```python
from build123d import *

# Parameters (mm, degrees)
EXTRUDE_1_DEPTH     = 22
EXTRUDE_2_DEPTH     = 21
CUT_EXTRUDE_1_REACH = 66.591
CUT_EXTRUDE_2_DEPTH = 11
FILLET_2_R          = 3
FILLET_3_R          = 4
SKETCH_6_W          = 11
SKETCH_6_H          = 2.5
EXTRUDE_6_DEPTH     = 5
FILLET_4_R          = 5
FILLET_5_R          = 2.5
SKETCH_7_R          = 1.5
CUT_EXTRUDE_3_DEPTH = 16
CUT_EXTRUDE_4_DEPTH = 11
CUT_EXTRUDE_5_DEPTH = 0.5
FILLET_7_R          = 1.5
FILLET_8_R          = 1
SKETCH_10_R         = 4.5
EXTRUDE_7_DEPTH     = 8
SKETCH_11_R         = 1.5
CUT_EXTRUDE_6_DEPTH = 3
CUT_EXTRUDE_START   = -3
SKETCH_12_R         = 1.5
CUT_EXTRUDE_7_DEPTH = 3


with BuildPart() as part:
    # Эскиз1 → Бобышка-Вытянуть1 (new, symmetric)
    with BuildSketch(Plane(origin=(0, 0, 0), x_dir=(0, 0, -1), z_dir=(1, 0, 0))):
        Polygon((0, -18), (0, 0), (58, 0), (58, -6), (2, -6), (2, -18), align=None)
    extrude(amount=EXTRUDE_1_DEPTH, both=True)

    # Эскиз2 → Бобышка-Вытянуть2 (add, symmetric)
    with BuildSketch(Plane(origin=(0, 0, 0), x_dir=(0, 0, -1), z_dir=(1, 0, 0))):
        Polygon((2, -6), (48, -6), (48, -7), (3, -7), (3, -17), (2, -17), align=None)
    extrude(amount=EXTRUDE_2_DEPTH, both=True)

    # Вырез-Вытянуть1: up to this face of the body (flat: up to its plane)
    cut_extrude_1_end = Plane(part.part.faces().sort_by_distance((0, -18, -1))[0])
    # Эскиз3 → Вырез-Вытянуть1 (cut, up to the picked face)
    with BuildSketch(Plane(origin=(0, 0, 0), x_dir=(1, 0, 0), z_dir=(0, 1, 0)), mode=Mode.PRIVATE) as cut_extrude_1_sk1:
        Polygon((-20, 58), (-22, 58), (-22, 0), align=None)
    cut_extrude_1_tool1 = split(extrude(cut_extrude_1_sk1.sketch, amount=-CUT_EXTRUDE_1_REACH, mode=Mode.PRIVATE), bisect_by=cut_extrude_1_end, keep=Keep.BOTH, mode=Mode.PRIVATE)
    # Эскиз3 → Вырез-Вытянуть1 (cut, up to the picked face)
    with BuildSketch(Plane(origin=(0, 0, 0), x_dir=(1, 0, 0), z_dir=(0, 1, 0)), mode=Mode.PRIVATE) as cut_extrude_1_sk2:
        Polygon((22, 58), (22, 0), (20, 58), align=None)
    cut_extrude_1_tool2 = split(extrude(cut_extrude_1_sk2.sketch, amount=-CUT_EXTRUDE_1_REACH, mode=Mode.PRIVATE), bisect_by=cut_extrude_1_end, keep=Keep.BOTH, mode=Mode.PRIVATE)
    add(cut_extrude_1_tool1.solids().sort_by(Axis((-21.333333, 0, -38.666667), (0, -1, 0)))[0], mode=Mode.SUBTRACT)
    add(cut_extrude_1_tool2.solids().sort_by(Axis((21.333333, 0, -38.666667), (0, -1, 0)))[0], mode=Mode.SUBTRACT)

    # Эскиз4 → Вырез-Вытянуть2 (cut)
    with BuildSketch(Plane.XZ.offset(6)):
        Polygon((-20.930440129, -2), (-19.344233233, -48), (-20.344827586, -48), (-21.931034483, -2), align=None)
        Polygon((19.344233233, -48), (20.344827586, -48), (21.931034483, -2), (20.930440129, -2), align=None)
    extrude(amount=CUT_EXTRUDE_2_DEPTH, mode=Mode.SUBTRACT)

    # Скругление2
    fillet_2_edges = [part.edges().sort_by_distance(p)[0] for p in [
        (19.344233233, -6.5, -48),
        (-19.344233233, -6.5, -48),
        (-20.91319875, -17, -2.5),
        (20.91319875, -17, -2.5),
    ]]
    fillet(fillet_2_edges, radius=FILLET_2_R)

    # Скругление3
    fillet_3_edges = [part.edges().sort_by_distance(p)[0] for p in [
        (-21.965517241, -18, -1),
        (21.965517241, -18, -1),
    ]]
    fillet(fillet_3_edges, radius=FILLET_3_R)

    # Эскиз6 → Бобышка-Вытянуть6 (add)
    with BuildSketch(Plane.XY):
        with Locations((-16.5, 1.25)):
            Rectangle(SKETCH_6_W, SKETCH_6_H)
        with Locations((16.5, 1.25)):
            Rectangle(SKETCH_6_W, SKETCH_6_H)
    extrude(amount=-EXTRUDE_6_DEPTH)

    # Скругление4
    fillet_4_edges = [part.edges().sort_by_distance(p)[0] for p in [
        (-20.913793103, 0, -31.5),
        (20.913793103, 0, -31.5),
    ]]
    fillet(fillet_4_edges, radius=FILLET_4_R)

    # Скругление5
    fillet_5_edges = [part.edges().sort_by_distance(p)[0] for p in [
        (-16.5, 2.5, -5),
        (-16.5, 2.5, 0),
        (16.5, 2.5, -5),
        (16.5, 2.5, 0),
    ]]
    fillet(fillet_5_edges, radius=FILLET_5_R - 0.0001)  # a hair under: the kernel refuses the full size

    # Эскиз7 → Вырез-Вытянуть3 (cut, symmetric)
    with BuildSketch(Plane(origin=(0, 0, 0), x_dir=(0, 0, -1), z_dir=(1, 0, 0))):
        with Locations((2.5, 0)):
            Circle(SKETCH_7_R)
    extrude(amount=CUT_EXTRUDE_3_DEPTH, both=True, mode=Mode.SUBTRACT)

    # Эскиз8 → Вырез-Вытянуть4 (cut, symmetric)
    with BuildSketch(Plane(origin=(0, 0, 0), x_dir=(0, 0, -1), z_dir=(1, 0, 0))):
        with BuildLine():
            Line((2.5, -2.5), (0, -2.5))
            Line((0, -2.5), (0, 0))
            ThreePointArc((0, 0), (4.267766953, 1.767766953), (2.5, -2.5))
        make_face()
    extrude(amount=CUT_EXTRUDE_4_DEPTH, both=True, mode=Mode.SUBTRACT)

    # Эскиз9 → Вырез-Вытянуть5 (cut)
    with BuildSketch(Plane(origin=(0, 0, -58), x_dir=(-1, 0, 0), z_dir=(0, 0, -1))):
        with BuildLine():
            Line((-14.997028232, -1), (14.997028232, -1))
            add(Edge.make_bspline(
                [(14.997028232, -1), (15.521093765, -1), (16.044951376, -1.104143211), (17.013235139, -1.504981238), (17.457278985, -1.801515154), (18.198254652, -2.542050681), (18.494897371, -2.985758471), (18.895847322, -3.953162299), (19, -4.476479025), (19, -5)],
                knots=[0, 0, 0, 0, 0.25, 0.25, 0.5, 0.5, 0.75, 0.75, 1, 1, 1, 1], degree=3))
            Line((19, -5), (19, -6))
            Line((19, -6), (-19, -6))
            Line((-19, -6), (-19, -5))
            add(Edge.make_bspline(
                [(-14.997028232, -1), (-15.521093765, -1), (-16.044951376, -1.104143211), (-17.013235139, -1.504981238), (-17.457278985, -1.801515154), (-18.198254652, -2.542050681), (-18.494897371, -2.985758471), (-18.895847322, -3.953162299), (-19, -4.476479025), (-19, -5)],
                knots=[0, 0, 0, 0, 0.25, 0.25, 0.5, 0.5, 0.75, 0.75, 1, 1, 1, 1], degree=3))
        make_face()
    extrude(amount=-CUT_EXTRUDE_5_DEPTH, mode=Mode.SUBTRACT)

    # Скругление7
    fillet_7_edges = [part.edges().sort_by_distance(p)[0] for p in [
        (0, -6, -57.5),
    ]]
    fillet(fillet_7_edges, radius=FILLET_7_R)

    # Скругление8
    fillet_8_edges = [part.edges().sort_by_distance(p)[0] for p in [
        (-19.5, -6, -58),
        (19.5, -6, -58),
    ]]
    fillet(fillet_8_edges, radius=FILLET_8_R)

    # Эскиз10 → Бобышка-Вытянуть7 (add, symmetric)
    with BuildSketch(Plane(origin=(0, 0, 0), x_dir=(0, 0, -1), z_dir=(1, 0, 0))):
        with Locations((58, -7)):
            Circle(SKETCH_10_R)
    extrude(amount=EXTRUDE_7_DEPTH, both=True)

    # Эскиз11 → Вырез-Вытянуть6 (cut)
    with BuildSketch(Plane(origin=(8, 0, 0), x_dir=(0, 0, -1), z_dir=(1, 0, 0))):
        with Locations((58, -7)):
            Circle(SKETCH_11_R)
    extrude(amount=-CUT_EXTRUDE_6_DEPTH, mode=Mode.SUBTRACT)

    # Эскиз12 → Вырез-Вытянуть7 (cut)
    with BuildSketch(Plane.ZY.offset(8).offset(CUT_EXTRUDE_START)):
        with Locations(Location((-58, -7, 0), (0, 0, 180))):
            Circle(SKETCH_12_R)
    extrude(amount=CUT_EXTRUDE_7_DEPTH, mode=Mode.SUBTRACT)

    # Эскиз13 → Вырез-Повернуть1 (revolve, cut)
    with BuildSketch(Plane(origin=(0, -7, 0), x_dir=(-1, 0, 0), z_dir=(0, 1, 0)), mode=Mode.PRIVATE) as cut_revolve_1_sk:
        with BuildLine():
            Line((-14.5, -58), (-8, -58))
            Line((-8, -58), (-8, -62.5))
            Line((-8, -62.5), (-10, -62.5))
            ThreePointArc((-10, -62.5), (-13.181980515, -61.181980515), (-14.5, -58))
        make_face()
        with BuildLine():
            Line((8, -58), (8, -62.5))
            Line((8, -62.5), (10, -62.5))
            ThreePointArc((10, -62.5), (13.181980515, -61.181980515), (14.5, -58))
            Line((14.5, -58), (8, -58))
        make_face()
    revolve(cut_revolve_1_sk.sketch.rotate(Axis((21.094367923, -7, -58), (-1, 0, 0)), 180), axis=Axis((21.094367923, -7, -58), (-1, 0, 0)), mode=Mode.SUBTRACT)


solid = part.part
```
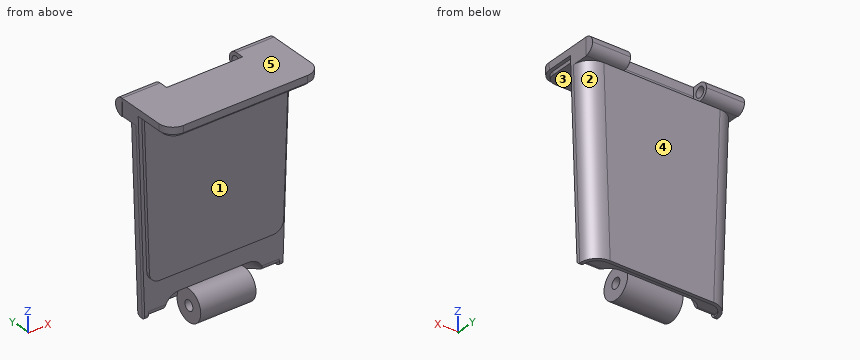
CAD build for the part. Positions are in the model's coordinates, mm. Face numbers are marked on the shaded views. A direction names the side the tool comes from. Round coordinates to 2 decimals unless told otherwise and drop trailing zeros. Order: outer loops, then holes, each group sorted by start corner. A loop starts at its lowest first (then second) coordinate and runs counter-clockwise, first axis right, second up.
Item 1: Pin check, flat tips, straight feed: pin 1 (1 mm diameter, centred on x = 10.5, z = -23, fed in from +Y); pin 2 (0.8 mm diameter, centred on x = 1, z = -2.5, fed in from -Y); pin 3 (6 mm diameter, centred on x = 6, y = -11.5, fed in from -Z); pin 4 (6 mm diameter, centred on y = -10.5, z = -29.5, fed in from +X). Stop position of each tip, or through.
Item 2: Saw through at C-C on y = -15.75. Write the cut outline in (x, z).
Item 3: Mould opens along Z. For the marked faces 3, 4 and 5 say: pulls with the +Z half, pulls with the -Z half, needs draft (parallel to the pull), parting line crosses it, or undercut.
Item 4: Tool access for the marked faces 1 and 2: list every direction of +Z, -Z, +X, -X, +Y, -Y with a clear straight run to the whole face (end or side of a thin tool).
Item 5: Probe line 1 along Y through (x, z) = (-13.8, -2.5); line 2 along Y through (x, z) = (8, -53); line 3 along Y through (x, z) = (17, -6). List the from-to ranges inside material, lowest first.
Item 6: Saw through at B-B on y = -9.75. Write the cut outline in (x, z).
Item 7: Saw through at D-D on x = -9. Write the cut outline in (y, z).
Item 8: Saw through at A-A on x = -3.5. Write the cut outline in (y, z), then the cut area to 3 significant figures.
Reported:
1. pin 1: stops at y = 0
1. pin 2: stops at y = -17
1. pin 3: stops at z = -62.24
1. pin 4: passes through
2. outline: (-21.6, 0) - (-21.53, -2) - (-20.37, -2) - (-20.33, -3) - (20.33, -3) - (20.37, -2) - (21.53, -2) - (21.6, 0) - close
3. face 3: undercut
3. face 4: needs draft
3. face 5: pulls with the +Z half
4. face 1: +X, -X, -Y
4. face 2: -Z, +X, +Y
5. line 1: y = -17 to -1.5, 1.5 to 2.5
5. line 2: y = -6 to 0
5. line 3: y = -7 to 0
6. outline: (-22, 0) - (-21.93, -2) - (-20.93, -2) - (-20.9, -3) - (20.9, -3) - (20.93, -2) - (21.93, -2) - (22, 0) - close; (-8, -61.56) - (8, -61.56) - (8, -54.44) - (-8, -54.44) - close
7. outline: (-18, -2) - (-17, -2) - (-17, -3) - (-7, -3) - (-7, -48) - (-6, -48) - (-6, -53.61) arc R4.5 cw to (-2.53, -57.5) - (-1, -57.5) - (-1, -58) - (0, -58) - (0, -5) arc R2.5 cw to (-2.5, -2.5) - (-2.5, 0) - (-18, 0) - close
8. outline: (-18, -2) - (-17, -2) - (-17, -3) - (-7, -3) - (-7, -48) - (-6, -48) - (-6, -53.61) arc R4.5 ccw (long way) to (-2.53, -57.5) - (-1, -57.5) - (-1, -58) - (0, -58) - (0, -5) arc R2.5 cw to (-2.5, -2.5) - (-2.5, 0) - (-18, 0) - close
8. area: 468 mm2
